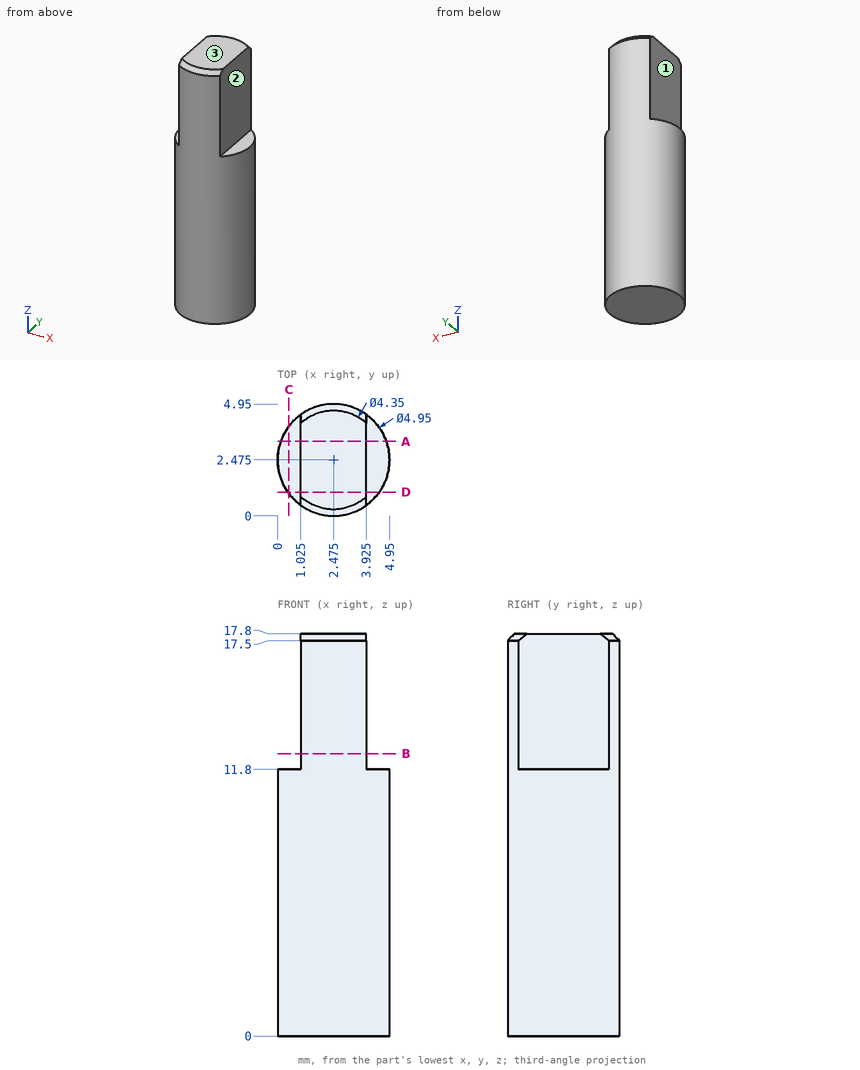
Study the drawing (mm; zero at the part's minimum x, y, z) and answer. A direction names the side the tool comes from. Round coordinates to 2 decimals unless told otherwise and drop trailing zeros. Write each loop counter-clockwise with the first axis right and the second up, starting at its lowest first coordinate (ties: lowest second). Pieces come first, ordered by that corner, then holes. Notation, with made-up numbers: (-17, 85) - (15, 85) arc R25 cw to (15, 98) - close; hole circle Ø2 at (-30, -21). An arc over 180 degrees is marked (long way). Return JSON: item names as keys, results as strings. Group by question number.
Q1. Find the intervals of material crossed by L1, parallel to X at y = 1.65, z = 15.75 (3 decimals); L2, parallel to Z at x = 4.3, y = 3.1; L3, parallel to Y at x = 2.35, z = 1.5, in increasing order.
Q2. The part is cut by section D-D on y = 1.05. Write down the section's boundary in (x, z) (3 decimals), then the cut area to 3 significant figures.
Q3. The part is cut by section B-B on z = 12.5. Write down the section's boundary in (x, y) (3 decimals), then the cut area to 3 significant figures.
Q4. The part is cut by section A-A on y = 3.3. Write down the section's boundary in (x, z) (3 decimals).
Q5. For the marked faces 1, 2 and 3, determine the directions among +Z, -Z, +X, -X, +Y, -Y from which every point of the face is accessible in a straight line to the end or side of a thin tool.
Q6. The part is cut by section C-C on x = 0.5. Write down the section's boundary in (y, z).
Q7. Each of these flat-tipped pins is pushed along its axis until it touches: pin 1 Ø1 at (y, z) = (2.5, 13.5) entering from -X (3 decimals); pin 2 Ø2 at (y, z) = (1, 3) entering from -X. Where does it stop, or does it pass through?
Solved:
{
 "1": {"L1": "1.025 to 3.925", "L2": "0 to 11.8", "L3": "0 to 4.95"},
 "2": {"outline": "(0.451, 0) - (4.499, 0) - (4.499, 11.8) - (3.925, 11.8) - (3.925, 17.8) - (1.025, 17.8) - (1.025, 11.8) - (0.451, 11.8) - close", "area": "65.2 mm²"},
 "3": {"outline": "(1.025, 0.469) arc R2.475 ccw to (3.925, 0.469) - (3.925, 4.481) arc R2.475 ccw to (1.025, 4.481) - close", "area": "13.5 mm²"},
 "4": {"outline": "(0.142, 0) - (4.808, 0) - (4.808, 11.8) - (3.925, 11.8) - (3.925, 17.8) - (1.025, 17.8) - (1.025, 11.8) - (0.142, 11.8) - close"},
 "5": {"face 1": "+Z, -X, +Y, -Y", "face 2": "+Z, +X, +Y, -Y", "face 3": "+Z, +X, -X, +Y, -Y"},
 "6": {"outline": "(0.98, 0) - (3.97, 0) - (3.97, 11.8) - (0.98, 11.8) - close"},
 "7": {"pin 1": "x = 1.025", "pin 2": "x = 0.05"}
}
